```python
from build123d import *

# Parameters (mm, degrees)
SKETCH1_R           = 27.325470016
BOSS_EXTRUDE1_DEPTH = 7.5
CUT_EXTRUDE1_DEPTH  = 7.5
CIRPATTERN1_COUNT   = 22


with BuildPart() as part:
    # Sketch1 → Boss-Extrude1 (new, symmetric)
    with BuildSketch(Plane.XY):
        Circle(SKETCH1_R)
    extrude(amount=BOSS_EXTRUDE1_DEPTH, both=True)

    # Sketch1_3 → Cut-Extrude1 (cut, symmetric)
    with BuildSketch(Plane.XY):
        with BuildLine():
            ThreePointArc((2.389000136, 26.557966834), (2.687762275, 27.004338738), (3.208387057, 27.136461893))
            ThreePointArc((3.208387057, 27.136461893), (-2.8e-08, 27.325470016), (-3.208387112, 27.136461887))
            ThreePointArc((-3.208387112, 27.136461887), (-2.687762323, 27.004338772), (-2.38900015, 26.557966895))
            ThreePointArc((-2.38900015, 26.557966895), (-3.2e-08, 24.651270016), (2.389000136, 26.557966834))
        make_face()
    cut_extrude1 = extrude(amount=CUT_EXTRUDE1_DEPTH, both=True, mode=Mode.SUBTRACT)

    # CirPattern1: Cut-Extrude1 ×22 about axis
    cirpattern1_axis = Axis((0, 0, 0), (0, 0, 1))
    for i in range(1, CIRPATTERN1_COUNT):
        add(cut_extrude1.rotate(cirpattern1_axis, i * 360 / CIRPATTERN1_COUNT), mode=Mode.SUBTRACT)


solid = part.part
```
The listing builds one solid part. Answer for the finished solid, in the listing's coordinates (mm). Round coordinates to 2 decimals unless told otherwise and drop trailing zeros. Write each loop counter-clockwise with the first axis right and the second up, starting at its lowest first coordinate (ties: lowest second). Pieces come first, ordered by that corner, then holes. Notation, with made-up numbers: (-34, 13.5) -> (5, 13.5) arc R12 cw to (5, 35.5) -> close; hole circle Ø5 at (63.25, 68). An arc over 180 degrees is marked (long way). Answer as a JSON object with one key per item and string values. Group by question number.
Q1. Determine the mould class of faces 1 (the face through (-0.05, 24.65, 0.11)), 2 (the face through (-13.289, -20.763, 0.105)), 3 (the face through (-26.22, -7.69, 0.11)) for opening direction Y: pulls with the +Y half, pulls with the -Y half, needs draft (parallel to the pull), parting line crosses it, or undercut.
Q2. Section A-A (y = -10) is taken. Write down the section's boundary in (x, z), plus the area to 4 significant figures.
Q3. Straight lines are drawn through the part: line 1 along X through (y, z) = (-11.5, 6.75); line 2 along X through (y, z) = (-4, 5.25); line 3 along Y through (x, z) = (7.5, -4.5). For each, find the intervals that lie inside material, in ascending order.
Q4. Each of these flat-tipped pins is pushed along its axis until it touches: pin 1 Ø4 at (y, z) = (14.5, 4.5) entering from +X; pin 2 Ø2 at (x, z) = (7, -6) entering from -Y; pin 3 Ø8 at (x, z) = (14, 3.5) entering from -Y. Where does it stop, or does it pass through?
Q5. Section B-B (x = 6.5) is taken. Write down the section's boundary in (y, z), plus the area to 3 significant figures.
Check values:
{
 "1": {"face 1": "pulls with the +Y half", "face 2": "undercut", "face 3": "pulls with the -Y half"},
 "2": {"outline": "(-22.55, -7.5) -> (22.55, -7.5) -> (22.55, 7.5) -> (-22.55, 7.5) -> close", "area": "676.5 mm^2"},
 "3": {"line 1": "-22.21 to 22.21", "line 2": "-24.38 to 24.38", "line 3": "-23.56 to 23.56"},
 "4": {"pin 1": "x = 23.46", "pin 2": "y = -24.18", "pin 3": "y = -25.19"},
 "5": {"outline": "(-23.83, -7.5) -> (23.83, -7.5) -> (23.83, 7.5) -> (-23.83, 7.5) -> close", "area": "715 mm^2"}
}
